Check sheet for the modelled part. Datum: model origin and axes. Units: mm. Face numbers are marked on the shaded views. A direction names the side the tool comes from. Round coordinates to 2 decimals unless told otherwise and drop trailing zeros. Order: outer loops, then holes, each group sorted by start corner. A loop starts at its lowest first (then second) coordinate and runs counter-clockwise, first axis right, second up. Notation, with made-up numbers: (-34, 1.5) -> (-29, 1.5) arc R23 ccw to (-29, 33.5) -> close; hole circle Ø1 at (29, 50.25). An arc over 180 degrees is marked (long way). Use CSV: the item, a comma, the result in double quotes.
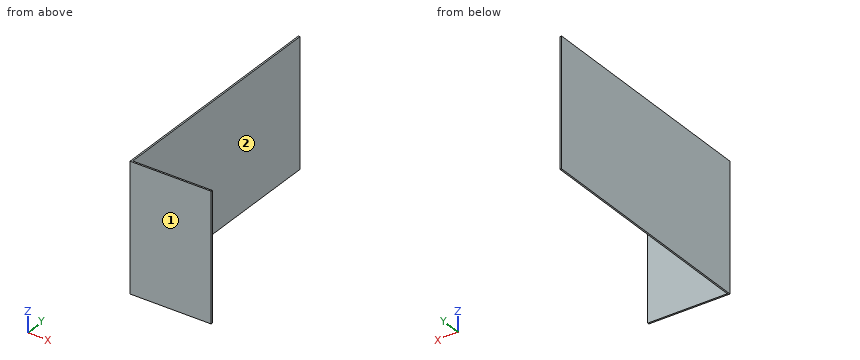
```python
from build123d import *

# Parameters (mm, degrees)
SKETCH1_W           = 50
SKETCH1_H           = 80
BOSS_EXTRUDE1_DEPTH = 1
SKETCH3_W           = 80
SKETCH3_H           = 150
BOSS_EXTRUDE2_DEPTH = 1


with BuildPart() as part:
    # Sketch1 → Boss-Extrude1 (new body)
    with BuildSketch(Plane(origin=(0, 0, 0), x_dir=(1, 0, 0), z_dir=(0, 1, 0))):
        Rectangle(SKETCH1_W, SKETCH1_H)
    extrude(amount=BOSS_EXTRUDE1_DEPTH)

    # Sketch3 → Boss-Extrude2 (add)
    with BuildSketch(Plane.ZY.offset(25)):
        with Locations((0, 75)):
            Rectangle(SKETCH3_W, SKETCH3_H)
    extrude(amount=BOSS_EXTRUDE2_DEPTH)


solid = part.part
```
Q1. Sectioned sample at A-A, the plane z = -9.5. Enter the section's corners in (x, y), then the cut area to 3 significant figures.
Result sheet:
outline,"(-26, 0) -> (25, 0) -> (25, 1) -> (-25, 1) -> (-25, 150) -> (-26, 150) -> close"
area,"200 mm^2"
Q2. Access from +Z, -Z, +X, -X, +Y, -Y to the whole of each face (thin tool, end or side, straight path). Record for the marked faces 1 and 2.
Result sheet:
face 1,"+Z, -Z, +X, -X, -Y"
face 2,"+Z, -Z, +X, +Y"
Q3. Go/stop test with flat-tipped pins: pin 1 (8 mm diameter, centred on x = -4, z = -15.5, fed in from +Y); pin 2 (1 mm diameter, centred on x = -1, z = -3.5, fed in from -Y). Record where each tip stops, or that it passes through.
Result sheet:
pin 1,"stops at y = 1"
pin 2,"stops at y = 0"
Q4. Sectioned sample at B-B, the plane x = 14. Enter the section's corners in (y, z), then the cut area to 3 significant figures.
Result sheet:
outline,"(0, -40) -> (1, -40) -> (1, 40) -> (0, 40) -> close"
area,"80.0 mm^2"
Q5. Scan lines: L1, parallel to Y at x = -20, z = -25.5; L2, parallel to X at y = 7, z = 19.5. Record each from-to range of solid material in increasing order.
Result sheet:
L1,"y = 0 to 1"
L2,"x = -26 to -25"
Q6. Sectioned sample at C-C, the plane y = 23. Enter the section's corners in (x, z), then the cut area to 3 significant figures.
Result sheet:
outline,"(-26, -40) -> (-25, -40) -> (-25, 40) -> (-26, 40) -> close"
area,"80.0 mm^2"
